The drawing under review shows one solid part. Ordinate dimensions are in mm from its lowest x, y, z. A direction names the side the tool comes from. Give positions to 0.01 mm unless a question says otherwise; leave off trailing zeros. Order: outer loops, then holes, each group sorted by start corner. A loop starts at its lowest first (then second) coordinate and runs counter-clockwise, first axis right, second up. Notation, with made-up numbers: (85.5, 41.25) - (100.5, 41.25) arc R24 ccw to (100.5, 71.25) - close; hole circle Ø3 at (79, 69). An arc over 180 degrees is marked (long way). Use CSV: the item, a comma, the result in double quotes. Start each with the question number.
1. Machinability: for the marked faces 5 and 6, which of the approach directions +Z, -Z, +X, -X, +Y, -Y give a long, thin tool a straight path to every point of the face, cutting with its end or side? Answer none if there is none.
2. For pin 1 (8 mm diameter, centred on x = 11, z = 20.5, fed in from -Y); pin 2 (3 mm diameter, centred on x = 18.5, z = 9, fed in from -Y) (1 decimal); pin 3 (6 mm diameter, centred on x = 21.5, z = 7, fed in from -Y), all flat-tipped, find the tip position at first contact; note any pin that passes through.
3. Take a section at B-B, the plane y = 18. State the section outline as (x, z) points, then the cut area to 3 significant figures.
4. To check wall thickness, follow line 1 (X direction, y = 17, z = 11.25) (1 decimal); line 2 (Y direction, x = 19.5, z = 5.75) (1 decimal); line 3 (Y direction, x = 4, z = 21). State the ranges of each line that lie inside material, in increasing order. Write a range as [from, to].
5. Take a section at A-A, the plane z = 15. State the section outline as (x, y) points.
6. Take a section at D-D, the plane x = 20. State the section outline as (y, z) points (1 decimal).
7. Take a section at C-C, the plane z = 4.5. State the section outline as (x, y) points.
8. Draft analysis for pull direction X (two halves, no side actions). For the marked faces 1, 2, 3 and 4, state which applies: released by +X, released by -X, zero draft, split by the parting line, or undercut.
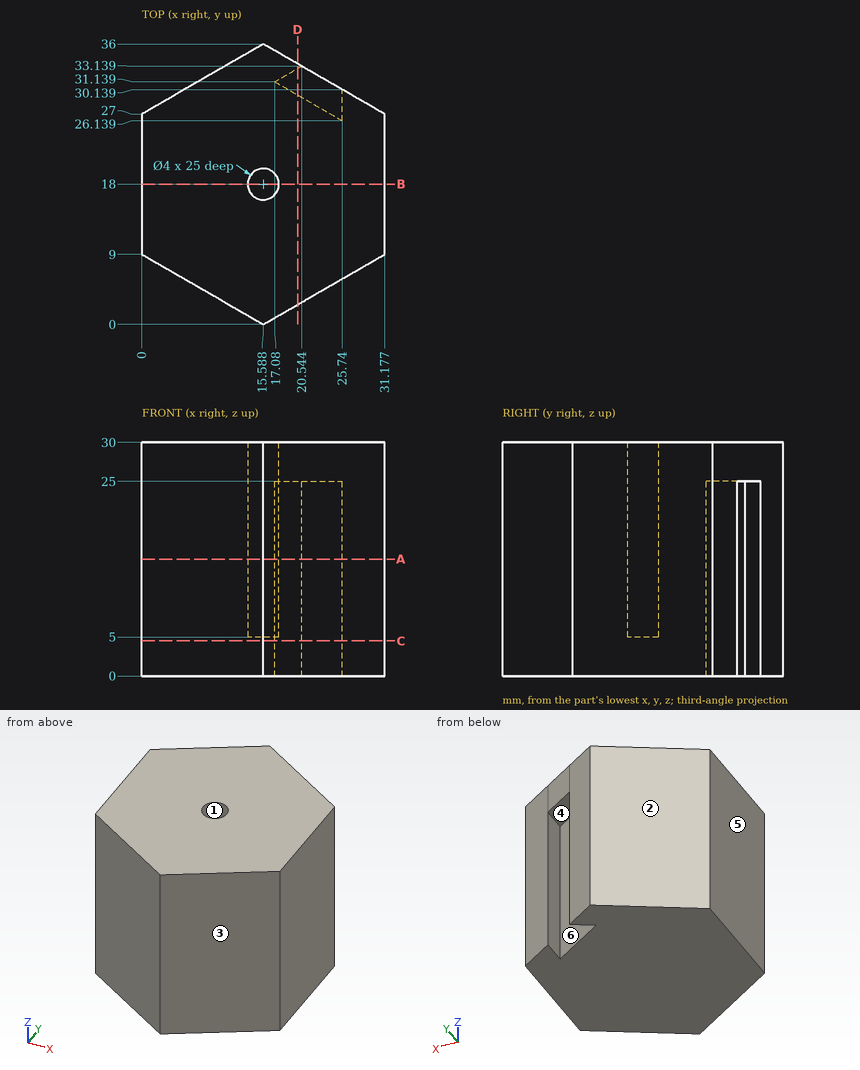
Determined:
1,face 5,"+Z, -Z, -X, +Y, -Y"
1,face 6,"-Z"
2,pin 1,"stops at y = 0.34"
2,pin 2,"stops at y = 0.8"
2,pin 3,"stops at y = 1.68"
3,outline,"(0, 0) - (31.18, 0) - (31.18, 30) - (17.59, 30) - (17.59, 5) - (13.59, 5) - (13.59, 30) - (0, 30) - close"
3,area,"835 mm²"
4,line 1,"x = [0, 13.9], [17.3, 31.2]"
4,line 2,"y = [2.3, 29.7], [32.5, 33.7]"
4,line 3,"y = [6.69, 29.31]"
5,outline,"(0, 9) - (15.59, 0) - (31.18, 9) - (31.18, 27) - (25.74, 30.14) - (25.74, 26.14) - (17.08, 31.14) - (20.54, 33.14) - (15.59, 36) - (0, 27) - close; hole circle Ø4 at (15.59, 18)"
6,outline,"(2.5, 0) - (29.5, 0) - (29.5, 25) - (32.8, 25) - (32.8, 0) - (33.5, 0) - (33.5, 30) - (2.5, 30) - close"
7,outline,"(0, 9) - (15.59, 0) - (31.18, 9) - (31.18, 27) - (25.74, 30.14) - (25.74, 26.14) - (17.08, 31.14) - (20.54, 33.14) - (15.59, 36) - (0, 27) - close"
8,face 1,"undercut"
8,face 2,"released by -X"
8,face 3,"released by +X"
8,face 4,"undercut"
